For this review, take the finished solid that the model builds, in its own axes (mm). Round coordinates to 2 decimals unless told otherwise and drop trailing zeros. Order: outer loops, then holes, each group sorted by start corner. A loop starts at its lowest first (then second) coordinate and runs counter-clockwise, first axis right, second up. Notation, with made-up numbers: (34, 49) - (71, 49) arc R16 cw to (71, 62) - close; hole circle Ø2 at (13, 7). An arc over 180 degrees is marked (long way). Write each question's results on one line, items separated by ' | '. Start each with the question number.
(1) Take a section at B-B, the plane y = 0.05. Give the boundary of the cut face in (x, z).
(2) Take a section at C-C, the plane z = 3.15. Give the boundary of the cut face in (x, y), plus the area to 3 significant figures.
(3) Take a section at A-A, the plane x = -2.4. Give the boundary of the cut face in (y, z).
(4) Take a section at D-D, the plane x = 2. Give the boundary of the cut face in (y, z).
(5) For L1, parallel to X at y = 2, z = 4.15; L2, parallel to Z at x = -1.9, y = -0.55; L3, parallel to Z at x = -0.95, y = 1.55, list the stretches that pass through material, from the lowest coordinate up. Write a range as from..to.
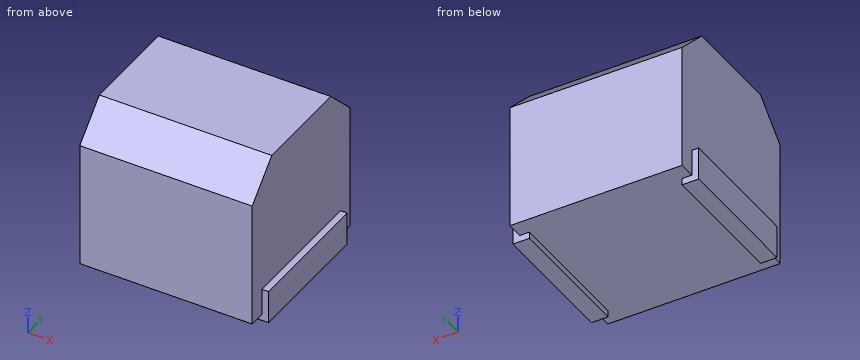
Autodesk Inventor part; units mm, degrees
ref_plane "YZ Plane" through (0, 0, 0) normal (1, 0, 0) x (0, 1, 0)
ref_plane "XZ Plane" through (0, 0, 0) normal (0, 1, 0) x (-1, 0, 0)
ref_plane "XY Plane" through (0, 0, 0) normal (0, 0, 1) x (1, 0, 0)
sketch "Sketch1" plane through (0, 0, 0) normal (0, 0, 1) x (1, 0, 0)
  line L0 (-2.8, 2.5) -> (2.8, 2.5)
  line L1 (2.8, 2.5) -> (2.8, -2.5)
  line L2 (2.8, -2.5) -> (-2.8, -2.5)
  line L3 (-2.8, -2.5) -> (-2.8, 2.5)
  line L4 (-2.8, 2.5) -> (2.8, -2.5) construction
  line L5 (2.8, 2.5) -> (-2.8, -2.5) construction
  point P0 (0, 0)
  dimension "d0" = 5.6
  dimension "d1" = 5
extrude "Extrusion1" add sketch "Sketch1" along normal blind 5
chamfer "Chamfer1" distance 1 angle 45 2 edges at (0, -2.5, 5) (0, 2.5, 5)
sketch "Sketch2" plane through (2.8, -2.5, 0) normal (1, 0, 0) x (0, 0, -1)
  line L0 (-5, 4) -> (-4, 5)
  line L1 (-5, 1) -> (-5, 4)
  line L2 (-4, 0) -> (-5, 1)
  line L3 (0, 0) -> (-4, 0)
  line L4 (0, 5) -> (0, 0)
  line L5 (0, 5) -> (-4, 5)
  line L6 (-1, 0.5) -> (0, 0.5)
  line L7 (0, 0.5) -> (0, 4.5)
  line L8 (0, 4.5) -> (-1, 4.5)
  line L9 (-1, 4.5) -> (-1, 0.5)
  point P0 (0, 2.5)
  dimension "d7" = 0.5
  dimension "d8" = 0.5
  dimension "d9" = 1
extrude "Extrusion2" cut sketch "Sketch2" against normal blind 0.2 contours L0 L5 L4 L8 L9 L6 L3 L2 L1
mirror "Mirror1" about plane through (0, 0, 0) normal (1, 0, 0) of "Extrusion2"
sketch "Sketch3" plane through (0, 0, 0) normal (0, 0, -1) x (-1, 0, 0)
  line L0 (2.6, -2.5) -> (2.6, -2)
  line L1 (2.6, -2) -> (2.8, -2)
  line L2 (2.8, -2) -> (2.8, 2)
  line L3 (2.8, 2) -> (2.6, 2)
  line L4 (2.6, 2) -> (2.6, 2.5)
  line L5 (2.6, 2.5) -> (-2.6, 2.5)
  line L6 (-2.6, 2.5) -> (-2.6, 2)
  line L7 (-2.6, 2) -> (-2.8, 2)
  line L8 (-2.8, 2) -> (-2.8, -2)
  line L9 (-2.8, -2) -> (-2.6, -2)
  line L10 (-2.6, -2) -> (-2.6, -2.5)
  line L11 (-2.6, -2.5) -> (2.6, -2.5)
  line L12 (2.8, -2) -> (2.3, -2)
  line L13 (2.3, -2) -> (2.3, 2)
  line L14 (2.3, 2) -> (2.8, 2)
  line L15 (2.8, 2) -> (2.8, -2)
  line L16 (-2.8, -2) -> (-2.3, -2)
  line L17 (-2.3, -2) -> (-2.3, 2)
  line L18 (-2.3, 2) -> (-2.8, 2)
  line L19 (-2.8, 2) -> (-2.8, -2)
  point P0 (0, 0)
  dimension "d12" = 0.5
  dimension "d13" = 4
  dimension "d14" = 0.5
  dimension "d15" = 4
extrude "Extrusion3" cut sketch "Sketch3" against normal blind 0.2 contours L11 L10 L16 L17 L18 L6 L5 L4 L14 L13 L12 L0
equation "\"d14\" = d12"
equation "\"d15\" = d13"
properties part number "NL565050T-103J-PF"
Results below:
1) outline: (-2.8, 0) - (-2.3, 0) - (-2.3, 0.2) - (2.3, 0.2) - (2.3, 0) - (2.8, 0) - (2.8, 1) - (2.6, 1) - (2.6, 5) - (-2.6, 5) - (-2.6, 1) - (-2.8, 1) - close
2) outline: (-2.6, -2.5) - (2.6, -2.5) - (2.6, 2.5) - (-2.6, 2.5) - close | area: 26.0 mm^2
3) outline: (-2.5, 0.2) - (-2, 0.2) - (-2, 0) - (2, 0) - (2, 0.2) - (2.5, 0.2) - (2.5, 4) - (1.5, 5) - (-1.5, 5) - (-2.5, 4) - close
4) outline: (-2.5, 0.2) - (2.5, 0.2) - (2.5, 4) - (1.5, 5) - (-1.5, 5) - (-2.5, 4) - close
5) L1: x = -2.6..2.6 | L2: z = 0.2..5 | L3: z = 0.2..4.95
